For this review, take the finished solid that the model builds, in its own axes (mm). A direction names the side the tool comes from. Coordinates: 2 decimals unless noted, no trailing zeros. Loops run counter-clockwise (first coordinate to the right, second up) from the corner with the lowest first, then second, coordinate; pieces in that order, holes last. Notation, with made-up numbers: M 77,68.25 L 111,68.25 A23 ccw 111,88.25 Z; hole C 78,41.5 d7. An arc over 180 degrees is marked long. Use one line per item in the form item = value.
```python
from build123d import *

# Parameters (mm, degrees)
ESQUISSE1_R        = 2.5
BOSS_EXTRU_1_DEPTH = 5
CONG_1_R           = 10


with BuildPart() as part:
    # Esquisse1 → Boss.-Extru.1 (new body)
    with BuildSketch(Plane.XY):
        Polygon((-40, 5), (-40, 0), (-40, -20), (-7.5, -62), (7.5, -62), (40, -20), (40, 0), (40, 5), (35, 5), (35, 0), (31.5, 0), (31.5, -3), (32.6, -3), (32.6, -5.3), (31.5, -5.3), (31.5, -10), (28.5, -10), (28.5, -5.3), (27.4, -5.3), (27.4, -3), (28.5, -3), (28.5, 0), (25, 0), (25, 5), (20, 5), (20, 0), (20, -20), (-20, -20), (-20, 0), (-20, 5), (-25, 5), (-25, 0), (-28.5, 0), (-28.5, -3), (-27.4, -3), (-27.4, -5.3), (-28.5, -5.3), (-28.5, -10), (-31.5, -10), (-31.5, -5.3), (-32.6, -5.3), (-32.6, -3), (-31.5, -3), (-31.5, 0), (-35, 0), (-35, 5), align=None)
        with Locations((0, -56)):
            Circle(ESQUISSE1_R, mode=Mode.SUBTRACT)
        with Locations((0, -26)):
            Circle(ESQUISSE1_R, mode=Mode.SUBTRACT)
    extrude(amount=BOSS_EXTRU_1_DEPTH)

    # Congé1
    cong_1_edges = [part.edges().sort_by_distance(p)[0] for p in [
        (-20, -20, 2.5),
        (20, -20, 2.5),
        (40, -20, 2.5),
        (7.5, -62, 2.5),
        (-7.5, -62, 2.5),
        (-40, -20, 2.5),
    ]]
    fillet(cong_1_edges, radius=CONG_1_R)


solid = part.part
```
1. For pin 1 Ø1.5 at (x, z) = (-30, 3.5) entering from +Y; pin 2 Ø12 at (x, y) = (-14, -52) entering from -Z; pin 3 Ø0.9 at (x, z) = (28, 2.5) entering from +Y; pin 4 Ø3 at (x, z) = (2.5, 1) entering from +Y, all flat-tipped, find the tip position at first contact; note any pin that passes through.
Computed values:
pin_1 = -10
pin_2 = 0
pin_3 = 0
pin_4 = -20
2. Consider section C-C on y = -26. Write out the cut boundary in (x, z).
Computed values:
outline = M -35.36,0 L -2.5,0 L -2.5,5 L -35.36,5 Z; M 2.5,0 L 35.36,0 L 35.36,5 L 2.5,5 Z
3. Consider section B-B on x = 0. Write out the cut boundary in (y, z).
Computed values:
outline = M -62,0 L -58.5,0 L -58.5,5 L -62,5 Z; M -53.5,0 L -28.5,0 L -28.5,5 L -53.5,5 Z; M -23.5,0 L -20,0 L -20,5 L -23.5,5 Z
4. Consider section D-D on z = 2.4. State how many separate pieces and enclosed holes the cut face has, plus the area to 3 significant figures.
Computed values:
separate_pieces = 1
enclosed_holes = 2
area = 2,820 mm2
5. Tool access review of faces 4 (the face through (6.941, -61.006, 2.535)), 5 (the face through (-25, 3, 2)), 6 (the face through (-32.6, -4, 2)): name each direction out of +Z, -Z, +X, -X, +Y, -Y from which nothing blocks a thin tool from reaching the whole face with its end or side.
Computed values:
face_4 = +Z, -Z, +X, -Y
face_5 = +Z, -Z, +Y
face_6 = +Z, -Z
6. Draft analysis for pull direction X (two halves, no side actions). For faces 1 (the face through (0, -20, 2)), 2 (the face through (-40, -6, 2)), 3 (the face through (23, 5, 2)), state which applies: +X half, -X half, draft (parallel to the pull), parting line (faces both ways), or undercut.
Computed values:
face_1 = undercut
face_2 = -X half
face_3 = draft
7. Consider section A-A on y = -1.5. Write out the cut boundary in (x, z), plus the area to 3 significant figures.
Computed values:
outline = M -40,0 L -31.5,0 L -31.5,5 L -40,5 Z; M -28.5,0 L -20,0 L -20,5 L -28.5,5 Z; M 20,0 L 28.5,0 L 28.5,5 L 20,5 Z; M 31.5,0 L 40,0 L 40,5 L 31.5,5 Z
area = 170 mm2
8. Wall thickness on line 1 along Y through (x, z) = (0, 2.6); line 2 along X through (y, z) = (-8, 2.95); line 3 along X through (y, z) = (-5, 3.65): over which ranges is each line inside the solid? List them lowest first. Write a range as from..to.
Computed values:
line_1 = -62..-58.5, -53.5..-28.5, -23.5..-20
line_2 = -40..-31.5, -28.5..-20, 20..28.5, 31.5..40
line_3 = -40..-32.6, -27.4..-20, 20..27.4, 32.6..40
